```python
from build123d import *

# Parameters (mm, degrees)
SKETCH1_R           = 20
BOSS_EXTRUDE1_DEPTH = 10
SKETCH2_W           = 35.08265457
SKETCH2_H           = 7.175997526
BOSS_EXTRUDE2_DEPTH = 30
FILLET1_R           = 5
SKETCH3_R           = 2.5
CUT_EXTRUDE1_DEPTH  = 30
SKETCH4_R           = 10
CUT_EXTRUDE2_DEPTH  = 5


with BuildPart() as part:
    # Sketch1 → Boss-Extrude1 (new body)
    with BuildSketch(Plane.XY):
        Circle(SKETCH1_R)
    extrude(amount=BOSS_EXTRUDE1_DEPTH)

    # Sketch2 → Boss-Extrude2 (add)
    with BuildSketch(Plane.XY.offset(10)):
        Rectangle(SKETCH2_W, SKETCH2_H)
    extrude(amount=BOSS_EXTRUDE2_DEPTH)

    # Fillet1
    fillet1_edges = [part.edges().sort_by_distance(p)[0] for p in [
        (17.541327285, 0, 40),
        (-17.541327285, 0, 40),
    ]]
    fillet(fillet1_edges, radius=FILLET1_R)

    # Sketch3 → Cut-Extrude1 (cut)
    with BuildSketch(Plane(origin=(0, 3.587998763, 0), x_dir=(1, 0, 0), z_dir=(0, 1, 0))):
        with Locations((-8.770663642, -28.75)):
            Circle(SKETCH3_R)
        with Locations((8.770663642, -28.75)):
            Circle(SKETCH3_R)
    extrude(amount=-CUT_EXTRUDE1_DEPTH, mode=Mode.SUBTRACT)

    # Sketch4 → Cut-Extrude2 (cut)
    with BuildSketch(Plane(origin=(0, 0, 0), x_dir=(-1, 0, 0), z_dir=(0, 0, -1))):
        Circle(SKETCH4_R)
    extrude(amount=-CUT_EXTRUDE2_DEPTH, mode=Mode.SUBTRACT)


solid = part.part
```
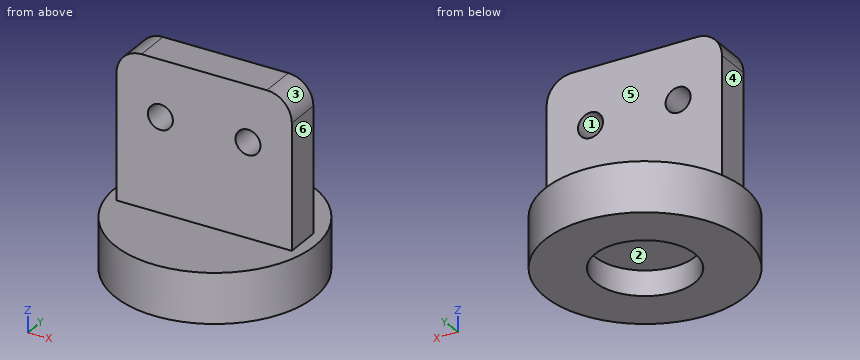
Could you check a few things on this model? Use its own coordinates, in mm. Face numbers are marked on the shaded views. A direction names the side the tool comes from. Give positions to 0.01 mm unless a question says otherwise; leave off trailing zeros. Loops run counter-clockwise (first coordinate to the right, second up) from the corner with the lowest first, then second, coordinate; pieces in that order, holes last. Notation, with made-up numbers: (68, 49.25) - (126, 49.25) arc R7 ccw to (126, 55.25) - close; hole circle Ø9 at (8, 45.25). An arc over 180 degrees is marked (long way). Answer in a Markdown table with one row per item. Add a question column.
Q1. Which directions (+Z, -Z, +X, -X, +Y, -Y) give clear straight access to the entire face, cutting with the end or side of a thin tool? Please do the marked faces 4, 5 and 6.
Q2. If we section it at D-D (x = 8): List the corners of the cut face in (y, z) for me, plus the area to 3 significant figures.
Q3. For pin 1 (2 mm diameter, centred on x = 5.5, z = 34.5, fed in from +Y); pin 2 (5 mm diameter, centred on x = -5.5, z = 30.5, fed in from -Y); pin 3 (2 mm diameter, centred on y = 1.5, z = 18, fed in from -X), each with a flat end and sliding along its axis, tell me the tip position at first contact or that it passes through.
Q4. We'd pull the mould along Z, two halves only. Please class the marked faces 1, 2 and 3: +Z half, -Z half, draft (parallel to the pull), parting line (faces both ways), or undercut.
Q5. Please list where these lines run through material, in increasing order: L1, parallel to X at y = -1.25, z = 28.75; L2, parallel to Y at x = 0, z = 2.55; L3, parallel to X at y = 0, z = 28. Write a range as from..to.
Q6. If we section it at A-A (z = 28.75): List the corners of the cut face in (x, y) for me, plus the area to 3 significant figures.
Q7. If we section it at C-C (x = 0): List the corners of the cut face in (y, z) for me, plus the area to 3 significant figures.
Q8. If we section it at B-B (y = 0): List the corners of the cut face in (x, z) for me, plus the area to 3 significant figures.
The answers:
| question | item | result |
|---|---|---|
| 1 | face 4 | +Z, -X, +Y, -Y |
| 1 | face 5 | +Z, +X, -X, +Y |
| 1 | face 6 | +Z, +X, +Y, -Y |
| 2 | outline | (-18.33, 0) - (-6, 0) - (-6, 5) - (6, 5) - (6, 0) - (18.33, 0) - (18.33, 10) - (3.59, 10) - (3.59, 26.37) - (-3.59, 26.37) - (-3.59, 10) - (-18.33, 10) - close; (-3.59, 31.13) - (3.59, 31.13) - (3.59, 40) - (-3.59, 40) - close |
| 2 | area | 488 mm^2 |
| 3 | pin 1 | stops at y = 3.59 |
| 3 | pin 2 | stops at y = -3.59 |
| 3 | pin 3 | stops at x = -17.54 |
| 4 | face 1 | undercut |
| 4 | face 2 | -Z half |
| 4 | face 3 | +Z half |
| 5 | L1 | x = -17.54..-11.27, -6.27..6.27, 11.27..17.54 |
| 5 | L2 | y = -20..-10, 10..20 |
| 5 | L3 | x = -17.54..-11.16, -6.39..6.39, 11.16..17.54 |
| 6 | outline | (-17.54, -3.59) - (-11.27, -3.59) - (-11.27, 3.59) - (-17.54, 3.59) - close; (-6.27, -3.59) - (6.27, -3.59) - (6.27, 3.59) - (-6.27, 3.59) - close; (11.27, -3.59) - (17.54, -3.59) - (17.54, 3.59) - (11.27, 3.59) - close |
| 6 | area | 180 mm^2 |
| 7 | outline | (-20, 0) - (-10, 0) - (-10, 5) - (10, 5) - (10, 0) - (20, 0) - (20, 10) - (3.59, 10) - (3.59, 40) - (-3.59, 40) - (-3.59, 10) - (-20, 10) - close |
| 7 | area | 515 mm^2 |
| 8 | outline | (-20, 0) - (-10, 0) - (-10, 5) - (10, 5) - (10, 0) - (20, 0) - (20, 10) - (17.54, 10) - (17.54, 35) arc R5 ccw to (12.54, 40) - (-12.54, 40) arc R5 ccw to (-17.54, 35) - (-17.54, 10) - (-20, 10) - close; hole circle Ø5 at (-8.77, 28.75); hole circle Ø5 at (8.77, 28.75) |
| 8 | area | 1,300 mm^2 |
